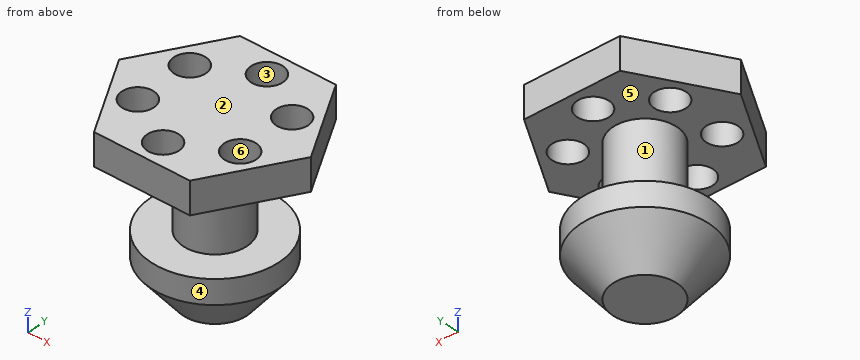
```python
from build123d import *

# Parameters (mm, degrees)
SKETCH1_R           = 12.7
BOSS_EXTRUDE3_DEPTH = 25.4


with BuildPart() as part:
    # Sketch1 → Boss-Extrude3 (new body)
    with BuildSketch(Plane.XY):
        Polygon((-76.2, 0), (-38.1, -65.991135768), (38.1, -65.991135768), (76.2, 0), (38.1, 65.991135768), (-38.1, 65.991135768), align=None)
        with Locations((0, -46.941135768)):
            Circle(SKETCH1_R, mode=Mode.SUBTRACT)
        with Locations((-40.652216058, -23.470567884)):
            Circle(SKETCH1_R, mode=Mode.SUBTRACT)
        with Locations((-40.652216058, 23.470567884)):
            Circle(SKETCH1_R, mode=Mode.SUBTRACT)
        with Locations((0, 46.941135768)):
            Circle(SKETCH1_R, mode=Mode.SUBTRACT)
        with Locations((40.652216058, 23.470567884)):
            Circle(SKETCH1_R, mode=Mode.SUBTRACT)
        with Locations((40.652216058, -23.470567884)):
            Circle(SKETCH1_R, mode=Mode.SUBTRACT)
    extrude(amount=BOSS_EXTRUDE3_DEPTH)

    # Sketch2 → Revolve-Thin1 (revolve)
    with BuildSketch(Plane(origin=(0, 0, 0), x_dir=(1, 0, 0), z_dir=(0, 1, 0))):
        Polygon((0, 0), (0, 114.3), (25.4, 114.3), (50.8, 82.55), (50.8, 63.5), (25.4, 63.5), (25.4, 0), (22.86, 0), (22.86, 66.04), (48.26, 66.04), (48.26, 81.659016109), (24.179212887, 111.76), (2.54, 111.76), (2.54, 0), align=None)
    revolve(axis=Axis((0, 0, -33.186581784), (0, 0, -1)))


solid = part.part
```
CAD build for the part. Positions are in the model's coordinates, mm. Face numbers are marked on the shaded views. A direction names the side the tool comes from. Give positions to 0.01 mm unless a question says otherwise; leave off trailing zeros. Order: outer loops, then holes, each group sorted by start corner. A loop starts at its lowest first (then second) coordinate and runs counter-clockwise, first axis right, second up.
(1) Saw through at A-A, the plane z = -72. Give the cut face in (x, y), then the cut area to 3 significant figures.
(2) Saw through at D-D, the plane z = -41. Give the cut face in (x, y), then the cut area to 3 significant figures.
(3) Tool access for the marked faces 4, 5 and 6: list every direction of +Z, -Z, +X, -X, +Y, -Y with a clear straight run to the whole face (end or side of a thin tool).
(4) Flat gauge pins, fed straight in: pin 1 (2 mm diameter, centred on y = 29.5, z = -84, fed in from -X); pin 2 (1 mm diameter, centred on x = 9.5, z = -57, fed in from -Y); pin 3 (23 mm diameter, centred on x = 40.65, y = -23.47, fed in from -Z). Where does each tip first touch, or does it go through?
(5) Mould opens along Y. For the marked faces 1, 2 and 3 say: released by +Y, released by -Y, zero draft, split by the parting line, or undercut.
(6) Drill centre lines: L1, parallel to X at y = 0, z = -73.75; L2, parallel to Y at x = 0, z = 9; L3, parallel to Y at x = -10, z = 8. Where is each one in solid material? Low to high.
(7) Saw through at B-B, the plane x = 0. State how many separate pieces and enclosed holes the cut face has, then the cut area to 3 significant figures.
(8) Saw through at C-C, the plane z = 15. Give the cut face in (x, y).
Results found:
1. outline: circle Ø101.6 at (0, 0); circle Ø5.08 at (0, 0); hole circle Ø96.52 at (0, 0)
1. area: 811 mm2
2. outline: circle Ø50.8 at (0, 0); circle Ø5.08 at (0, 0); hole circle Ø45.72 at (0, 0)
2. area: 405 mm2
3. face 4: -Z
3. face 5: none
3. face 6: +Z
4. pin 1: stops at x = -41.14
4. pin 2: stops at y = -23.75
4. pin 3: stops at z = -101.75
5. face 1: split by the parting line
5. face 2: zero draft
5. face 3: undercut
6. L1: x = -50.8 to -48.26, -2.54 to 2.54, 48.26 to 50.8
6. L2: y = -65.99 to -59.64, -34.24 to 34.24, 59.64 to 65.99
6. L3: y = -65.99 to -54.77, -39.11 to 39.11, 54.77 to 65.99
7. separate pieces: 3
7. enclosed holes: 2
7. area: 3,500 mm2
8. outline: (-76.2, 0) - (-38.1, -65.99) - (38.1, -65.99) - (76.2, 0) - (38.1, 65.99) - (-38.1, 65.99) - close; hole circle Ø25.4 at (-40.65, -23.47); hole circle Ø25.4 at (-40.65, 23.47); hole circle Ø25.4 at (0, -46.94); hole circle Ø25.4 at (0, 46.94); hole circle Ø25.4 at (40.65, -23.47); hole circle Ø25.4 at (40.65, 23.47)
